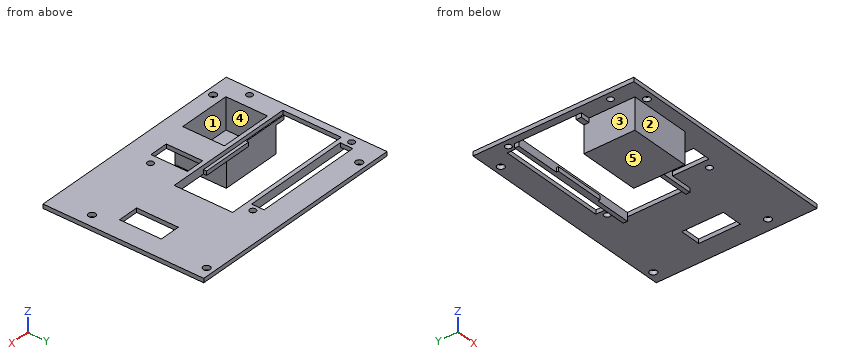
```python
from build123d import *

# Parameters (mm, degrees)
SKETCH_W      = 107.5
SKETCH_H      = 77.1
SKETCH_R      = 1.7
SKETCH_R_2    = 1.5
SKETCH_W_2    = 63.7
SKETCH_H_2    = 28
SKETCH_W_3    = 25.3
SKETCH_H_3    = 20
SKETCH_W_4    = 52
SKETCH_H_4    = 6
SKETCH_W_5    = 10
SKETCH_W_6    = 9
SKETCH_H_5    = 17.5
PAD_DEPTH     = 2
PAD003_DEPTH  = 2
SKETCH005_W   = 29.3
SKETCH005_H   = 24.5
SKETCH005_W_2 = 25.3
SKETCH005_H_2 = 20
PAD004_DEPTH  = 13
SKETCH006_W   = 29.3
SKETCH006_H   = 24.5
PAD005_DEPTH  = 2


with BuildPart() as part:
    # Sketch (on XY_Plane of Origin) → Pad (new body)
    with BuildSketch(Plane.XY):
        with Locations((53.75, 38.55)):
            Rectangle(SKETCH_W, SKETCH_H)
        with Locations((12, 73.6)):
            Circle(SKETCH_R, mode=Mode.SUBTRACT)
        with Locations((12, 3.5)):
            Circle(SKETCH_R, mode=Mode.SUBTRACT)
        with Locations((101.5, 73.6)):
            Circle(SKETCH_R, mode=Mode.SUBTRACT)
        with Locations((101.5, 18.6)):
            Circle(SKETCH_R, mode=Mode.SUBTRACT)
        with Locations((61.5, 63)):
            Circle(SKETCH_R_2, mode=Mode.SUBTRACT)
        with Locations((61.5, 14)):
            Circle(SKETCH_R_2, mode=Mode.SUBTRACT)
        with Locations((3.5, 14)):
            Circle(SKETCH_R_2, mode=Mode.SUBTRACT)
        with Locations((3.5, 63)):
            Circle(SKETCH_R_2, mode=Mode.SUBTRACT)
        with Locations((35.35, 44)):
            Rectangle(SKETCH_W_2, SKETCH_H_2, mode=Mode.SUBTRACT)
        with Locations((22.65, 18)):
            Rectangle(SKETCH_W_3, SKETCH_H_3, mode=Mode.SUBTRACT)
        with Locations((32.5, 63)):
            Rectangle(SKETCH_W_4, SKETCH_H_4, mode=Mode.SUBTRACT)
        with Locations((92.5, 38.55)):
            Rectangle(SKETCH_W_5, SKETCH_H_3, mode=Mode.SUBTRACT)
        with Locations((52.5, 19.25)):
            Rectangle(SKETCH_W_6, SKETCH_H_5, mode=Mode.SUBTRACT)
    extrude(amount=PAD_DEPTH)

    # Sketch004 → Pad003 (join)
    with BuildSketch(Plane(origin=(0, 0, 0), x_dir=(1, 0, 0), z_dir=(0, 0, -1))):
        Polygon((3.5, -58), (3.5, -60), (67.2, -60), (67.2, -58), (50, -58), (50, -57), (25.5, -57), (25.5, -58), align=None)
        Polygon((67.2, -30), (67.2, -28), (3.5, -28), (3.5, -30.5), (25.5, -30.5), (25.5, -31.5), (50, -31.5), (50, -30), align=None)
    extrude(amount=PAD003_DEPTH)

    # Sketch005 (on Face4 of Pad003) → Pad004 (join)
    with BuildSketch(Plane(origin=(0, 0, 0), x_dir=(1, 0, 0), z_dir=(0, 0, -1))):
        with Locations((22.65, -18.25)):
            Rectangle(SKETCH005_W, SKETCH005_H)
        with Locations((22.65, -18)):
            Rectangle(SKETCH005_W_2, SKETCH005_H_2, mode=Mode.SUBTRACT)
    extrude(amount=PAD004_DEPTH)

    # Sketch006 (on Face48 of Pad004) → Pad005 (join)
    with BuildSketch(Plane(origin=(0, 0, -13), x_dir=(1, 0, 0), z_dir=(0, 0, -1))):
        with Locations((22.65, -18.25)):
            Rectangle(SKETCH006_W, SKETCH006_H)
    extrude(amount=PAD005_DEPTH)


solid = part.part
```
CAD build for the part. Positions are in the model's coordinates, mm. Face numbers are marked on the shaded views. A direction names the side the tool comes from. Round coordinates to 2 decimals unless told otherwise and drop trailing zeros. Order: outer loops, then holes, each group sorted by start corner. A loop starts at its lowest first (then second) coordinate and runs counter-clockwise, first axis right, second up. Notation, with made-up numbers: (-35.5, 9.25) - (-20.5, 9.25) arc R17 ccw to (-20.5, 29.25) - close; hole circle Ø6 at (-9.5, -31.75). An arc over 180 degrees is marked (long way). Use CSV: the item, a comma, the result in double quotes. Start each with the question number.
1) Saw through at C-C (z = -5.25). List the corners of the cut face in (x, y), and give its area (3 significant figures).
2) Saw through at A-A (y = 43.5). List the corners of the cut face in (x, z).
3) Saw through at D-D (y = 3.5). List the corners of the cut face in (x, z), and give its area (3 significant figures).
4) Wall check: L1, parallel to X at y = 73.6, z = 1.65; L2, parallel to Y at x = 12, z = 0.8; L3, parallel to Y at x = 61.5, z = 1.5. Give the ranges that are in metal, low to high. Write a range as [from, to].
5) Two-plate mould, pull along Y, no slides. Class the marked faces 1, 2 and 3: pulls with the +Y half, pulls with the -Y half, needs draft (parallel to the pull), parting line crosses it, or undercut.
6) Saw through at B-B (x = 54). List the corners of the cut face in (y, z).
7) Pin check, flat tips, straight feed: pin 1 Ø6 at (x, z) = (24, -8) entering from -Y; pin 2 Ø2.5 at (x, y) = (3.5, 14) entering from +Z; pin 3 Ø4 at (x, y) = (101.5, 18.6) entering from -Z; pin 4 Ø12 at (x, y) = (31.5, 54) entering from +Z. Stop position of each tip, or through.
8) Tool access for the marked faces 4 and 5: list every direction of +Z, -Z, +X, -X, +Y, -Y with a clear straight run to the whole face (end or side of a thin tool).
Values follow:
1,outline,"(8, 6) - (37.3, 6) - (37.3, 30.5) - (8, 30.5) - close; hole (10, 8) - (35.3, 8) - (35.3, 28) - (10, 28) - close"
1,area,"212 mm2"
2,outline,"(0, 0) - (3.5, 0) - (3.5, 2) - (0, 2) - close; (67.2, 0) - (87.5, 0) - (87.5, 2) - (67.2, 2) - close; (97.5, 0) - (107.5, 0) - (107.5, 2) - (97.5, 2) - close"
3,outline,"(0, 0) - (10.3, 0) - (10.3, 2) - (0, 2) - close; (13.7, 0) - (107.5, 0) - (107.5, 2) - (13.7, 2) - close"
3,area,"208 mm2"
4,L1,"x = [0, 10.3], [13.7, 99.8], [103.2, 107.5]"
4,L2,"y = [0, 1.8], [5.2, 8], [28, 30], [58, 60], [66, 71.9], [75.3, 77.1]"
4,L3,"y = [0, 12.5], [15.5, 30], [58, 61.5], [64.5, 77.1]"
5,face 1,"undercut"
5,face 2,"pulls with the -Y half"
5,face 3,"needs draft"
6,outline,"(0, 0) - (10.5, 0) - (10.5, 2) - (0, 2) - close; (28, -2) - (30, -2) - (30, 2) - (28, 2) - close; (58, -2) - (60, -2) - (60, 2) - (58, 2) - close; (66, 0) - (77.1, 0) - (77.1, 2) - (66, 2) - close"
7,pin 1,"stops at y = 6"
7,pin 2,"passes through"
7,pin 3,"stops at z = 0"
7,pin 4,"stops at z = 2"
8,face 4,"+Z"
8,face 5,"-Z, +X, -X, +Y, -Y"
